from build123d import *

# Parameters (mm, degrees)
CROQUIS1_RX             = 85
CROQUIS1_RY             = 67.73101263
SALIENTE_EXTRUIR1_DEPTH = 200
CORTAR_EXTRUIR1_DEPTH   = 100
SALIENTE_EXTRUIR2_DEPTH = 30
CROQUIS5_R              = 7.5
SALIENTE_EXTRUIR3_DEPTH = 30
CORTAR_EXTRUIR3_DEPTH   = 30
CROQUIS8_W              = 78.88877914
CROQUIS8_H              = 202.201910825
CORTAR_EXTRUIR4_DEPTH   = 348.816388214
CROQUIS9_R              = 15
CORTAR_EXTRUIR5_DEPTH   = 20
CROQUIS10_R             = 7.5
CORTAR_EXTRUIR6_DEPTH   = 8
CORTAR_EXTRUIR7_DEPTH   = 12.5


with BuildPart() as part:
    # Croquis1 → Saliente-Extruir1 (new body)
    with BuildSketch(Plane.XY):
        with Locations(Location((-119.067557665, 97.160736636), (0, 0, 90))):
            Ellipse(CROQUIS1_RX, CROQUIS1_RY)
    extrude(amount=SALIENTE_EXTRUIR1_DEPTH)

    # Croquis3 → Cortar-Extruir1 (cut)
    with BuildSketch(Plane.XY.offset(200)):
        with BuildLine():
            Line((-171.829854236, 137.159885706), (-171.829854236, 57.159885706))
            Line((-171.829854236, 57.159885706), (-178.829854236, 57.159885706))
            add(Edge.make_bspline(
                [(-178.830577491, 137.159885706), (-195.829371976, 97.159643663), (-178.829854236, 57.159885706)],
                knots=[1.080850346, 1.080850346, 1.080850346, 2.060764999, 2.060764999, 2.060764999], degree=2, weights=[1, 0.882352941, 1]))
            Line((-178.830577491, 137.159885706), (-171.829854236, 137.159885706))
        make_face()
    extrude(amount=-CORTAR_EXTRUIR1_DEPTH, mode=Mode.SUBTRACT)

    # Croquis4 → Saliente-Extruir2 (add)
    with BuildSketch(Plane.XY.offset(200)):
        with BuildLine():
            Line((-178.830577491, 137.159885706), (-171.829854236, 137.159885706))
            Line((-171.829854236, 137.159885706), (-171.829854236, 57.159885706))
            Line((-171.829854236, 57.159885706), (-178.829854236, 57.159885706))
            add(Edge.make_bspline(
                [(-178.830577491, 137.159885706), (-195.797797403, 97.186782087), (-178.829854236, 57.159885706)],
                knots=[4.219557052, 4.219557052, 4.219557052, 5.198274326, 5.198274326, 5.198274326], degree=2, weights=[1, 0.882634519, 1]))
        make_face()
    extrude(amount=-SALIENTE_EXTRUIR2_DEPTH)

    # Croquis5 → Saliente-Extruir3 (add)
    with BuildSketch(Plane(origin=(0, 0, 0), x_dir=(-1, 0, 0), z_dir=(0, 0, -1))):
        with Locations(Location((119.067557665, 97.160736636, 0), (0, 0, 180))):
            Circle(CROQUIS5_R)
    extrude(amount=SALIENTE_EXTRUIR3_DEPTH)

    # Croquis7 → Cortar-Extruir3 (cut)
    with BuildSketch(Plane.XY.offset(200)):
        with BuildLine():
            Line((-131.567557665, 42.160736636), (-106.567557665, 42.160736636))
            Line((-106.567557665, 42.160736636), (-106.567557665, 13.620827843))
            add(Edge.make_bspline(
                [(-131.567557665, 13.620827843), (-119.067557665, 10.675126293), (-106.567557665, 13.620827843)],
                knots=[6.0975677, 6.0975677, 6.0975677, 6.468802915, 6.468802915, 6.468802915], degree=2, weights=[1, 0.982822456, 1]))
            Line((-131.567557665, 13.620827843), (-131.567557665, 42.160736636))
        make_face()
        with BuildLine():
            Line((-131.567557665, 180.700645429), (-131.567557665, 152.160736636))
            Line((-131.567557665, 152.160736636), (-106.567557665, 152.160736636))
            Line((-106.567557665, 152.160736636), (-106.567557665, 180.700645429))
            add(Edge.make_bspline(
                [(-106.567557665, 180.700645429), (-119.067557665, 183.64634698), (-131.567557665, 180.700645429)],
                knots=[2.955975046, 2.955975046, 2.955975046, 3.327210261, 3.327210261, 3.327210261], degree=2, weights=[1, 0.982822456, 1]))
        make_face()
    extrude(amount=-CORTAR_EXTRUIR3_DEPTH, mode=Mode.SUBTRACT)

    # Croquis8 → Cortar-Extruir4 (cut, through all)
    with BuildSketch(Plane.XY.offset(200)):
        with Locations((-158.511947235, 101.100955412)):
            Rectangle(CROQUIS8_W, CROQUIS8_H)
    extrude(amount=-CORTAR_EXTRUIR4_DEPTH, mode=Mode.SUBTRACT)

    # Croquis9 → Cortar-Extruir5 (cut)
    with BuildSketch(Plane.XY.offset(200)):
        with Locations((-119.067557665, 97.160736636)):
            Circle(CROQUIS9_R)
    extrude(amount=-CORTAR_EXTRUIR5_DEPTH, mode=Mode.SUBTRACT)

    # Croquis10 → Cortar-Extruir6 (cut)
    with BuildSketch(Plane.ZY.offset(106.567557665)):
        with Locations((185, 169.660736636)):
            Circle(CROQUIS10_R)
        with Locations((185, 24.660736636)):
            Circle(CROQUIS10_R)
    extrude(amount=-CORTAR_EXTRUIR6_DEPTH, mode=Mode.SUBTRACT)

    # Croquis11 → Cortar-Extruir7 (cut)
    with BuildSketch(Plane.ZY.offset(119.067557665)):
        Polygon((170, 152.160736636), (81.545095526, 184.35568894), (86.604252386, 216.899683734), (170, 209.051385078), align=None)
        Polygon((170, 42.160736636), (54.164328104, 0), (170, 0), align=None)
    extrude(amount=-CORTAR_EXTRUIR7_DEPTH, mode=Mode.SUBTRACT)


solid = part.part
Model file for the job. Use its own axes, mm. A direction names the side the tool comes from. Give positions to 0.01 mm unless a question says otherwise; leave off trailing zeros.
Item 1: Drill centre lines: line 1 along Y through (x, z) = (-101.25, 185); line 2 along Z through (x, y) = (-107, 63); line 3 along Z through (x, y) = (-101, 20.5). Where is each one in solid material? Low to high.
Check values:
line 1: y = 15.15 to 17.16, 32.16 to 162.16, 177.16 to 179.17
line 2: z = 0 to 200
line 3: z = 0 to 178.76, 191.24 to 200
Item 2: Which spindle directions (+Z, -Z, +X, -X, +Y, -Y) get a long thin tool onto all of the face, cutting with end or side? Do faces 1 (the face through (-113, 152.161, 185)), 2 (the face through (-98.568, 170, 185)), 3 (the face through (-111.57, 97.33, -14.79)), 4 (the face through (-106.568, 25, 159)), 5 (the face through (-113, 97, 180)). Say none if no direction does.
Check values:
face 1: +Z, -X, +Y
face 2: -X
face 3: -Z, +X
face 4: +Z, -X, -Y
face 5: +Z, -X
Item 3: Mould opens along Y. For faces 6 (the face through (-85, 98, 200)), 7 (the face through (-102.624, 171.914, 192.154)), 8 (the face through (-112.91, 27.37, 129.36)) say: +Y half, -Y half, draft (parallel to the pull), parting line (faces both ways), or undercut.
Check values:
face 6: draft
face 7: undercut
face 8: -Y half
Item 4: Drop flat-ended pins along their axis: P1, Ø6.5, axis at x = -110.5, z = 187, coming from the -Y side; P2, Ø23, axis at y = 24.5, z = 173, coming from the -X side; P3, Ø1.5, axis at y = 40.5, z = 39.5, coming from the +X side; P4, Ø8, axis at x = -84, z = -5.5, coming from the -Y side. Give the stop position or say it passes through.
Check values:
P1: stops at y = 42.16
P2: stops at x = -106.57
P3: stops at x = -68.05
P4: passes through
